Read the model definition and answer for the solid it produces. Units are mm, in the model's axes. Face numbers are marked on the shaded views. A direction names the side the tool comes from. Coordinates: 2 decimals unless noted, no trailing zeros. Write each loop counter-clockwise with the first axis right and the second up, starting at its lowest first coordinate (ties: lowest second). Pieces come first, ordered by that corner, then holes. Notation, with made-up numbers: (-10, -2) - (-6, -2) arc R14 ccw to (-6, 10) - close; hole circle Ø11 at (82, -38). An arc over 180 degrees is marked (long way). Return JSON: item names as keys, results as strings.
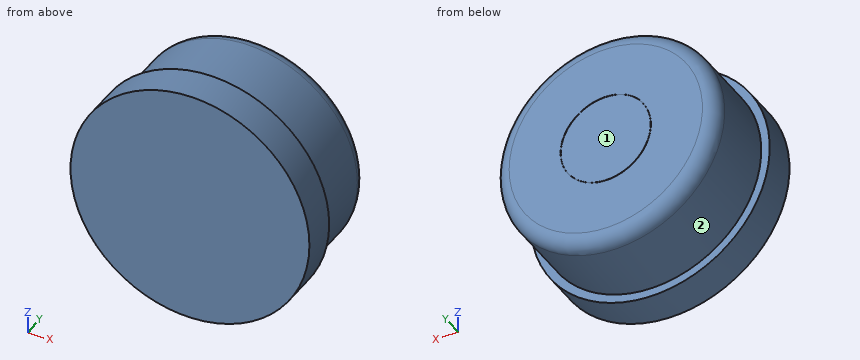
```python
from build123d import *

# Parameters (mm, degrees)
SKETCH1_R               = 8.4455
BOSS_EXTRUDE1_DEPTH     = 2.54
SKETCH2_R               = 7.8486
BOSS_EXTRUDE2_DEPTH     = 8.255
FILLET1_R               = 1.016
SKETCH3_R               = 3.2004
SKETCH3_R_2             = 3.175
CUT_EXTRUDE_THIN1_DEPTH = 0.0254


with BuildPart() as part:
    # Sketch1 → Boss-Extrude1 (new body)
    with BuildSketch(Plane(origin=(0, 0, 0), x_dir=(1, 0, 0), z_dir=(0, 1, 0))):
        Circle(SKETCH1_R)
    extrude(amount=BOSS_EXTRUDE1_DEPTH)

    # Sketch2 → Boss-Extrude2 (add)
    with BuildSketch(Plane(origin=(0, 0, 0), x_dir=(1, 0, 0), z_dir=(0, 1, 0))):
        Circle(SKETCH2_R)
    extrude(amount=BOSS_EXTRUDE2_DEPTH)

    # Fillet1
    fillet1_edges = [part.edges().sort_by_distance(p)[0] for p in [
        (-7.8486, 8.255, 0),
    ]]
    fillet(fillet1_edges, radius=FILLET1_R)

    # Sketch3 → Cut-Extrude-Thin1 (cut)
    with BuildSketch(Plane(origin=(0, 8.255, 0), x_dir=(1, 0, 0), z_dir=(0, 1, 0))):
        Circle(SKETCH3_R)
        Circle(SKETCH3_R_2, mode=Mode.SUBTRACT)
    extrude(amount=-CUT_EXTRUDE_THIN1_DEPTH, mode=Mode.SUBTRACT)


solid = part.part
```
(1) A cutting plane is placed at C-C (y = 0.5). Determine the outline of the cut face in (x, z), and give its area (3 significant figures).
Answer:
{"outline": "circle Ø16.89 at (0, 0)", "area": "224 mm²"}
(2) A cutting plane is placed at D-D (y = 6.5). Determine the outline of the cut face in (x, z), and give its area (3 significant figures).
Answer:
{"outline": "circle Ø15.7 at (0, 0)", "area": "194 mm²"}
(3) Which of the six approach directions +Z, -Z, +X, -X, +Y, -Y give full straight-line access (tool end or side, diameter ignored) to the marked faces 1 and 2?
Answer:
{"face 1": "+Z, -Z, +X, -X, +Y", "face 2": "+Y"}
(4) Straight lines are drawn through the part: line 1 (Y direction, x = 7.75, z = 3.25); line 2 (Y direction, x = 5.25, z = 4.5); line 3 (X direction, y = 3, z = 3.5) (3 decimals). For each, find the intervals that lie inside material, in ascending order. Write a range as from..to.
Answer:
{"line 1": "0..2.54", "line 2": "0..8.25", "line 3": "-7.025..7.025"}
